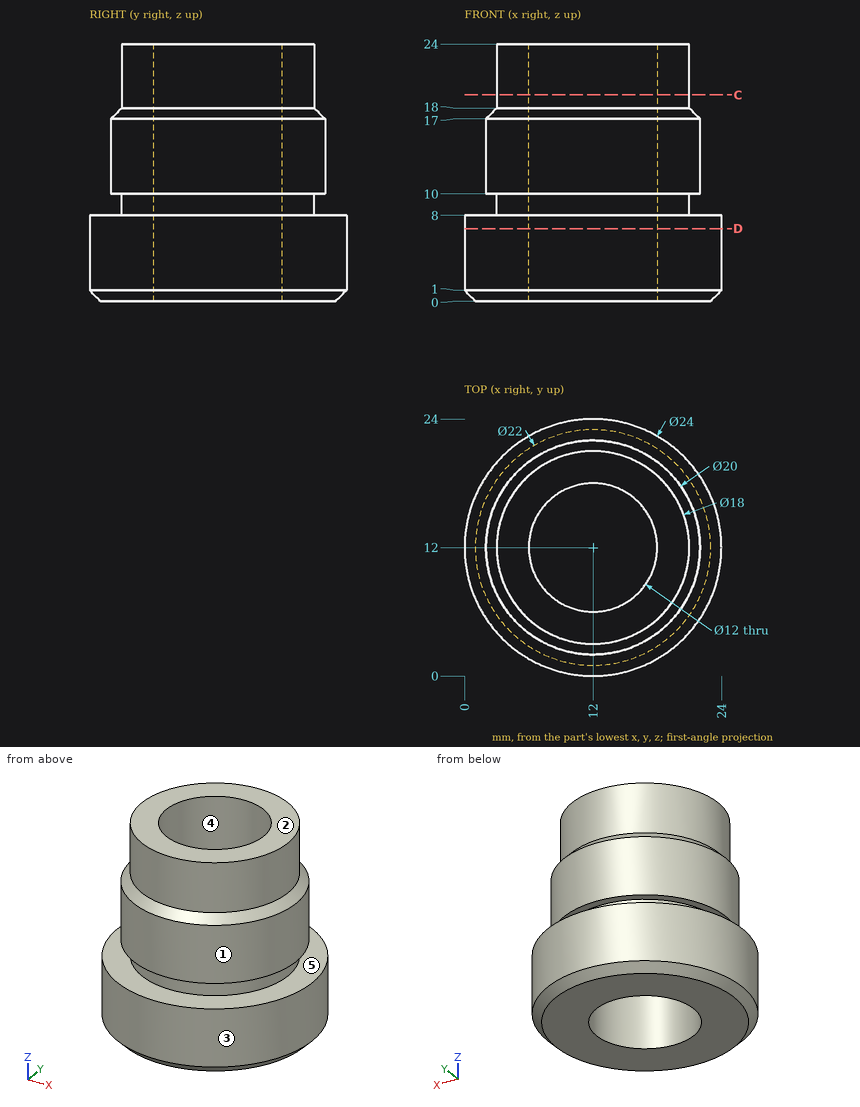
The drawing under review shows one solid part. Ordinate dimensions are in mm from its lowest x, y, z. A direction names the side the tool comes from. Give positions to 0.01 mm unless a question says otherwise; leave off trailing zeros. Loops run counter-clockwise (first coordinate to the right, second up) from the corner with the lowest first, then second, coordinate; pieces in that order, holes last. Notation, with made-up numbers: M 63,89.25 L 96,89.25 A28 cw 96,122.25 Z; hole C 53,-23 d3. An arc over 180 degrees is marked long. One line per item, written item: value. Start each with the question number.
Q1. Add section D-D (z = 6.75). Give the boundary of the cut face in (x, y).
Q2. For L1, parallel to Y at x = 12, z = 6.5; L2, parallel to Y at x = 12, z = 15.5; L3, parallel to X at y = 13.25, z = 4.5, list the stretches that pass through material, from the lowest coordinate up.
Q3. Clearance check with flat-ended pins moving along their axes: pin 1 Ø1.5 at (x, z) = (20.5, 15.5) entering from -Y; pin 2 Ø10 at (y, z) = (5, 6.5) entering from +X; pin 3 Ø12 at (y, z) = (3.5, 15) entering from -X. State where each tip first meets the part, or that it passes through.
Q4. Draft analysis for pull direction X (two halves, no side actions). For the marked faces 3, 4 and 5, state which applies: released by +X, released by -X, zero draft, split by the parting line, or undercut.
Q5. Machinability: for the marked faces 1 and 2, which of the approach directions +Z, -Z, +X, -X, +Y, -Y give a long, thin tool a straight path to every point of the face, cutting with its end or side? Answer none if there is none.
Q6. Add section C-C (z = 19.25). Give the boundary of the cut face in (x, y), and give its area (3 significant figures).
Reply:
1. outline: C 12,12 d24; hole C 12,12 d12
2. L1: 0 to 6, 18 to 24
2. L2: 2 to 6, 18 to 22
2. L3: 0.07 to 6.13, 17.87 to 23.93
3. pin 1: y = 5.68
3. pin 2: x = 23.83
3. pin 3: x = 2.32
4. face 3: split by the parting line
4. face 4: undercut
4. face 5: zero draft
5. face 1: +Z
5. face 2: +Z, +X, -X, +Y, -Y
6. outline: C 12,12 d18; hole C 12,12 d12
6. area: 141 mm²
